from build123d import *

# Parameters (mm, degrees)
SKETCH_1_W           = 40
SKETCH_1_H           = 70
SKETCH_1_R           = 4
EXTRUDE_1_DEPTH      = 10
SKETCH_2_W           = 5
SKETCH_2_H           = 22
CUT_EXTRUDE_1_DEPTH  = 55.083269132
SKETCH_3_R           = 7.5
EXTRUDE_2_DEPTH      = 18
SKETCH_4_R           = 10
EXTRUDE_3_DEPTH      = 2
EXTRUDE_4_DEPTH      = 1.5
EXTRUDE_4_DEPTH_BACK = 1.5
SKETCH_6_R           = 5
CUT_EXTRUDE_2_DEPTH  = 50.081564767
SKETCH_7_R           = 10
SKETCH_7_R_2         = 7.5
CUT_EXTRUDE_3_DEPTH  = 48.968739821


with BuildPart() as part:
    # Эскиз1 → Бобышка-Вытянуть1 (new body)
    with BuildSketch(Plane.XY):
        Rectangle(SKETCH_1_W, SKETCH_1_H)
        with Locations((13, -28)):
            Circle(SKETCH_1_R, mode=Mode.SUBTRACT)
        with Locations((-13, -28)):
            Circle(SKETCH_1_R, mode=Mode.SUBTRACT)
        with BuildLine():
            Line((10, 21), (10, 28))
            ThreePointArc((10, 28), (13, 31), (16, 28))
            Line((16, 28), (16, 21))
            ThreePointArc((16, 21), (13, 18), (10, 21))
        make_face(mode=Mode.SUBTRACT)
        with BuildLine():
            Line((-16, 21), (-16, 28))
            ThreePointArc((-16, 28), (-13, 31), (-10, 28))
            Line((-10, 28), (-10, 21))
            ThreePointArc((-10, 21), (-13, 18), (-16, 21))
        make_face(mode=Mode.SUBTRACT)
    extrude(amount=EXTRUDE_1_DEPTH)

    # Эскиз2 → Вырез-Вытянуть1 (cut, through all)
    with BuildSketch(Plane(origin=(20, 0, 0), x_dir=(0, 0, -1), z_dir=(1, 0, 0))):
        with Locations((-2.5, 24)):
            Rectangle(SKETCH_2_W, SKETCH_2_H)
    extrude(amount=-CUT_EXTRUDE_1_DEPTH, mode=Mode.SUBTRACT)

    # Эскиз3 → Бобышка-Вытянуть2 (add)
    with BuildSketch(Plane.XY.offset(10)):
        with Locations(Location((0, 0, 0), (0, 0, 180))):
            Circle(SKETCH_3_R)
    extrude(amount=EXTRUDE_2_DEPTH)

    # Эскиз4 → Бобышка-Вытянуть3 (add)
    with BuildSketch(Plane.XY.offset(28)):
        Circle(SKETCH_4_R)
    extrude(amount=-EXTRUDE_3_DEPTH)

    # Эскиз5 → Бобышка-Вытянуть4 (add, two sides: drawn at the far end of the back side and taken through both)
    with BuildSketch(Plane(origin=(0, 0, 0), x_dir=(0, 0, -1), z_dir=(1, 0, 0)).offset(-EXTRUDE_4_DEPTH_BACK)):
        Polygon((-10, 35), (-28, 0), (-10, -35), align=None)
    extrude(amount=EXTRUDE_4_DEPTH + EXTRUDE_4_DEPTH_BACK)

    # Эскиз6 → Вырез-Вытянуть2 (cut, through all)
    with BuildSketch(Plane.XY.offset(28)):
        Circle(SKETCH_6_R)
    extrude(amount=-CUT_EXTRUDE_2_DEPTH, mode=Mode.SUBTRACT)

    # Эскиз7 → Вырез-Вытянуть3 (cut, through all)
    with BuildSketch(Plane(origin=(0, 0, 26), x_dir=(-1, 0, 0), z_dir=(0, 0, -1))):
        Circle(SKETCH_7_R)
        Circle(SKETCH_7_R_2, mode=Mode.SUBTRACT)
    extrude(amount=-CUT_EXTRUDE_3_DEPTH, mode=Mode.SUBTRACT)


solid = part.part
The listing builds one solid part. Answer for the finished solid, in the listing's coordinates (mm). A direction names the side the tool comes from. Round coordinates to 2 decimals unless told otherwise and drop trailing zeros. Write each loop counter-clockwise with the first axis right and the second up, starting at its lowest first coordinate (ties: lowest second). Pieces come first, ordered by that corner, then holes. Notation, with made-up numbers: (2.5, -28.75) - (32.5, -28.75) arc R21 ccw to (32.5, -8.75) - close; hole circle Ø3 at (19, 24). An arc over 180 degrees is marked (long way). Use a Markdown table: item, result. Add a question column.
1. For a pull along Y with two mould halves and no side action, classify faces 4 (the face through (11, 0, 10)), 5 (the face through (-16, 24, 7)), 6 (the face through (0, -21, 17.2)) as +Y half, -Y half, draft (parallel to the pull), parting line (faces both ways), or undercut.
2. The part is cut by section D-D (z = 2.75). Write down the section's boundary in (x, y).
3. A tool of negligible diameter and unlimited length cuts with its end or side. For faces 1 (the face through (0, 24, 5)), 2 (the face through (10, 24, 7)), 3 (the face through (-3.461, 6.654, 18.874)), from which of +Z, -Z, +X, -X, +Y, -Y can it reach the whole face along a straight path? Write none if from no direction.
4. The part is cut by section C-C (y = -28). Write down the section's boundary in (x, z), and give its area (3 significant figures).
5. Consider line 1 (Y direction, x = -13, z = 7); line 2 (Y direction, x = -13, z = 2.5); line 3 (Z direction, x = -5.5, y = 19.5). Determine where each line is inside the solid, lowest interval first.
6. The part is cut by section A-A (y = 0). Write down the section's boundary in (x, z).
7. Flat-ended cylindrical pins translate along their axes: P1, Ø3, axis at y = 17, z = 20, coming from the +X side; P2, Ø2, axis at y = -6, z = 20.5, coming from the -X side; P3, Ø17.5, axis at x = 3, y = 27, coming from the -Z side. Find the tip coordinate at first contact, or state that the pin passes through.
8. The part is cut by section B-B (x = 13). Write down the section's boundary in (y, z), and give its area (3 significant figures).
Reported:
| question | item | result |
|---|---|---|
| 1 | face 4 | draft |
| 1 | face 5 | undercut |
| 1 | face 6 | -Y half |
| 2 | outline | (-20, -35) - (20, -35) - (20, 13) - (-20, 13) - close; hole circle Ø8 at (-13, -28); hole circle Ø10 at (0, 0); hole circle Ø8 at (13, -28) |
| 3 | face 1 | -Z, +X, -X, +Y |
| 3 | face 2 | +Z, -Z |
| 3 | face 3 | +Z |
| 4 | outline | (-20, 0) - (-17, 0) - (-17, 10) - (-20, 10) - close; (-9, 0) - (9, 0) - (9, 10) - (1.5, 10) - (1.5, 13.6) - (-1.5, 13.6) - (-1.5, 10) - (-9, 10) - close; (17, 0) - (20, 0) - (20, 10) - (17, 10) - close |
| 4 | area | 251 mm^2 |
| 5 | line 1 | -35 to -32, -24 to 18, 31 to 35 |
| 5 | line 2 | -35 to -32, -24 to 13 |
| 5 | line 3 | 5 to 10 |
| 6 | outline | (-20, 0) - (-5, 0) - (-5, 28) - (-7.5, 28) - (-7.5, 10) - (-20, 10) - close; (5, 0) - (20, 0) - (20, 10) - (7.5, 10) - (7.5, 28) - (5, 28) - close |
| 7 | P1 | x = 1.5 |
| 7 | P2 | x = -5.59 |
| 7 | P3 | z = 5 |
| 8 | outline | (-35, 0) - (-32, 0) - (-32, 10) - (-35, 10) - close; (-24, 0) - (13, 0) - (13, 5) - (18, 5) - (18, 10) - (-24, 10) - close; (31, 5) - (35, 5) - (35, 10) - (31, 10) - close |
| 8 | area | 445 mm^2 |
